For this review, take the finished solid that the model builds, in its own axes (mm). Give positions to 0.01 mm unless a question says otherwise; leave off trailing zeros. Loops run counter-clockwise (first coordinate to the right, second up) from the corner with the lowest first, then second, coordinate; pieces in that order, holes last. Notation, with made-up numbers: (-21, 68.25) - (38, 68.25) arc R18 ccw to (38, 77.25) - close; hole circle Ø5 at (30.25, -15). An arc over 180 degrees is marked (long way). Put each result on its own line as item: value.
from build123d import *

# Parameters (mm, degrees)
ESQUISSE1_R        = 15
BOSS_EXTRU_1_DEPTH = 10


with BuildPart() as part:
    # Esquisse1 → Boss.-Extru.1 (new body)
    with BuildSketch(Plane.XY):
        with BuildLine():
            Line((0, 0), (0, 170))
            Line((0, 170), (15.883900487, 213.64065792))
            ThreePointArc((15.883900487, 213.64065792), (44.814020761, 239.011692472), (81.755876566, 228.244123434))
            Line((81.755876566, 228.244123434), (90, 220))
            Line((90, 220), (140, 170))
            Line((140, 170), (310, 0))
            Line((310, 0), (0, 0))
        make_face()
        with Locations((52.354231449, 205)):
            Circle(ESQUISSE1_R, mode=Mode.SUBTRACT)
    extrude(amount=BOSS_EXTRU_1_DEPTH)


solid = part.part
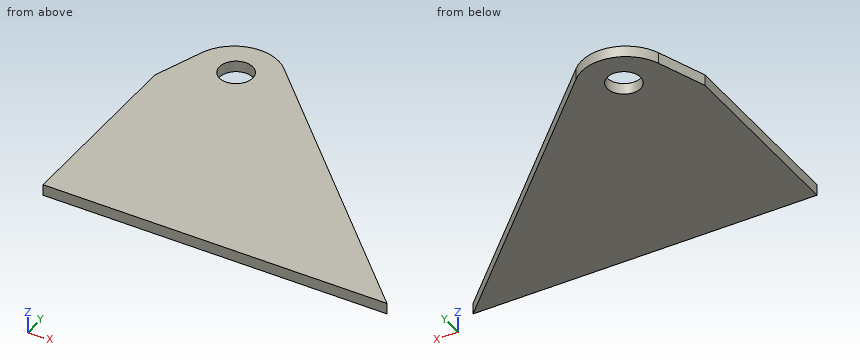
1) Take a section at D-D on x = 194. State the section outline as (y, z) points.
Geometry check:
outline: (0, 0) - (116, 0) - (116, 10) - (0, 10) - close
2) Insertion check: pin 1 Ø1 at (y, z) = (201.5, 2.5) entering from -X; pin 2 Ø5 at (x, z) = (104, 6.5) entering from +Y. Each pin has a flat end and moves straight along its axis. Give the tip position at first contact, or say it passes through.
Geometry check:
pin 1: stops at x = 11.28
pin 2: stops at y = 208.5
3) Wall thickness on line 1 (X direction, y = 90, z = 4.75); line 2 (Y direction, x = 62, z = 4.5); line 3 (Y direction, x = 216, z = 8): over which ranges is each line inside the solid? List them lowest first.
Geometry check:
line 1: x = 0 to 220
line 2: y = 0 to 193.51, 216.49 to 239.04
line 3: y = 0 to 94
4) Take a section at A-A on z = 2.5. State the section outline as (x, y) points, and give its area (3 significant figures).
Geometry check:
outline: (0, 0) - (310, 0) - (81.76, 228.24) arc R40 ccw to (15.88, 213.64) - (0, 170) - close; hole circle Ø30 at (52.35, 205)
area: 43,800 mm²
5) Take a section at B-B on y = 205. State the section outline as (x, z) points.
Geometry check:
outline: (12.74, 0) - (37.35, 0) - (37.35, 10) - (12.74, 10) - close; (67.35, 0) - (105, 0) - (105, 10) - (67.35, 10) - close
6) Take a section at C-C on x = 53.5. State the section outline as (y, z) points, and give its area (3 significant figures).
Geometry check:
outline: (0, 0) - (190.04, 0) - (190.04, 10) - (0, 10) - close; (219.96, 0) - (239.96, 0) - (239.96, 10) - (219.96, 10) - close
area: 2,100 mm²
